```python
from build123d import *

# Parameters (mm, degrees)
SKETCH_1_W                         = 60
SKETCH_1_H                         = 20
SM_BASE_FLANGE_1_DEPTH             = 2
SM_EDGE_FLANGE_1_STRIP_W           = 13.4732
SM_EDGE_FLANGE_1_STRIP_H           = 2
SM_EDGE_FLANGE_1_STRIP_CUT_DEPTH   = 20
SM_EDGE_FLANGE_1_STRIP_2_W         = 13.4732
SM_EDGE_FLANGE_1_STRIP_2_H         = 2
SM_EDGE_FLANGE_1_STRIP_CUT_2_DEPTH = 20
SM_EDGE_FLANGE_1_DEPTH             = 20
SM_EDGE_FLANGE_1_BEND_DEPTH        = 20
SM_EDGE_FLANGE_1_PROFILE_W         = 45
SM_EDGE_FLANGE_1_PROFILE_H         = 17.2634
SM_EDGE_FLANGE_1_FLAT_DEPTH        = 2
RIB_2_REACH                        = 74.312
SKETCH_12_WALL_W                   = 160.765785142
SKETCH_12_WALL_H                   = 3
CUT_EXTRUDE_1_REACH                = 86.433
SKETCH_13_R                        = 2.75
CUT_EXTRUDE_1_DIRECTION_2_DEPTH    = 85.433405711
SKETCH_15_R                        = 2.75
CUT_EXTRUDE_2_DEPTH                = 10
SKETCH_16_R                        = 2.25
CUT_EXTRUDE_3_DEPTH                = 10


# Sheet-metal steps are written as plain solids
with BuildPart() as part:
    # Sketch 1 → 基体-法兰1 (new body)
    with BuildSketch(Plane(origin=(0, 0, 0), x_dir=(1, 0, 0), z_dir=(0, 1, 0))):
        Rectangle(SKETCH_1_W, SKETCH_1_H)
    extrude(amount=-SM_BASE_FLANGE_1_DEPTH)

    # 边线-法兰1 strip (across the edge) → 边线-法兰1 strip cut (cut)
    with BuildSketch(Plane(origin=(30, 0, 10), x_dir=(-1, 0, 0), z_dir=(0, 0, -1))):
        with Locations((-2, -1)):
            Rectangle(SM_EDGE_FLANGE_1_STRIP_W, SM_EDGE_FLANGE_1_STRIP_H)
    extrude(amount=SM_EDGE_FLANGE_1_STRIP_CUT_DEPTH, mode=Mode.SUBTRACT)

    # 边线-法兰1 strip 2 (across the edge) → 边线-法兰1 strip cut 2 (cut)
    with BuildSketch(Plane(origin=(-30, 0, -10), x_dir=(1, 0, 0), z_dir=(0, 0, 1))):
        with Locations((-2, -1)):
            Rectangle(SM_EDGE_FLANGE_1_STRIP_2_W, SM_EDGE_FLANGE_1_STRIP_2_H)
    extrude(amount=SM_EDGE_FLANGE_1_STRIP_CUT_2_DEPTH, mode=Mode.SUBTRACT)

    # 边线-法兰1 section (across the edge) → 边线-法兰1 (add)
    with BuildSketch(Plane(origin=(30, 0, 10), x_dir=(-1, 0, 0), z_dir=(0, 0, -1))):
        with BuildLine():
            Line((0, 2.7366), (0, 48))
            Line((0, 48), (2, 48))
            Line((2, 48), (2, 2.7366))
            ThreePointArc((2, 2.7366), (2.801531583, 0.801531583), (4.7366, 0))
            Line((4.7366, 0), (4.7366, -2))
            ThreePointArc((4.7366, -2), (1.38731802, -0.61268198), (0, 2.7366))
        make_face()
    extrude(amount=SM_EDGE_FLANGE_1_DEPTH)

    # 边线-法兰1 bend section (across the edge) → 边线-法兰1 bend (add)
    with BuildSketch(Plane(origin=(-30, 0, -10), x_dir=(1, 0, 0), z_dir=(0, 0, 1))):
        with BuildLine():
            Line((0, 2.7366), (2, 2.7366))
            ThreePointArc((2, 2.7366), (2.801531583, 0.801531583), (4.7366, 0))
            Line((4.7366, 0), (4.7366, -2))
            ThreePointArc((4.7366, -2), (1.38731802, -0.61268198), (0, 2.7366))
        make_face()
    extrude(amount=SM_EDGE_FLANGE_1_BEND_DEPTH)

    # 边线-法兰1 profile (on flange) → 边线-法兰1 flat (add)
    with BuildSketch(Plane(origin=(-30, 0, 0), x_dir=(0, 0, -1), z_dir=(1, 0, 0))):
        with Locations((-12.5, 11.3683)):
            Rectangle(SM_EDGE_FLANGE_1_PROFILE_W, SM_EDGE_FLANGE_1_PROFILE_H)
    extrude(amount=SM_EDGE_FLANGE_1_FLAT_DEPTH)

    # 草图12 wall → 筋2 (add, up to next)
    with BuildSketch(Plane(origin=(-23, 5, -10), x_dir=(0.707106781187, -0.707106781187, 0), z_dir=(-0.707106781187, -0.707106781187, 0)), mode=Mode.PRIVATE) as rib_2_sk1:
        with Locations((0, 1.5)):
            Rectangle(SKETCH_12_WALL_W, SKETCH_12_WALL_H)
    rib_2_tool1 = extrude(rib_2_sk1.sketch, amount=RIB_2_REACH, mode=Mode.PRIVATE) - part.part
    rib_2 = rib_2_tool1.solids().sort_by_distance((-23, 5, -10))[0]
    add(rib_2)

    # 镜向1: 筋2 across plane
    add(rib_2.mirror(Plane(origin=(0, 0, 0), x_dir=(0, 0, 1), z_dir=(1, 0, 0))))

    # 草图13 → 切除-拉伸1 (cut, up to next)
    with BuildSketch(Plane.ZY.offset(30), mode=Mode.PRIVATE) as cut_extrude_1_sk1:
        with Locations(Location((0, 13, 0), (0, 0, 90))):
            Circle(SKETCH_13_R)
    cut_extrude_1_tool1 = extrude(cut_extrude_1_sk1.sketch, amount=-CUT_EXTRUDE_1_REACH, mode=Mode.PRIVATE) & part.part
    # 草图13 → 切除-拉伸1 (cut, up to next)
    with BuildSketch(Plane.ZY.offset(30), mode=Mode.PRIVATE) as cut_extrude_1_sk2:
        with Locations(Location((19, 13, 0), (0, 0, 90))):
            Circle(SKETCH_13_R)
    cut_extrude_1_tool2 = extrude(cut_extrude_1_sk2.sketch, amount=-CUT_EXTRUDE_1_REACH, mode=Mode.PRIVATE) & part.part
    # 草图13 → 切除-拉伸1 (cut, up to next)
    with BuildSketch(Plane.ZY.offset(30), mode=Mode.PRIVATE) as cut_extrude_1_sk3:
        with Locations(Location((30, 13, 0), (0, 0, 90))):
            Circle(SKETCH_13_R)
    cut_extrude_1_tool3 = extrude(cut_extrude_1_sk3.sketch, amount=-CUT_EXTRUDE_1_REACH, mode=Mode.PRIVATE) & part.part
    add(cut_extrude_1_tool1.solids().sort_by_distance((-30, 13, 0))[0], mode=Mode.SUBTRACT)
    add(cut_extrude_1_tool2.solids().sort_by_distance((-30, 13, 19))[0], mode=Mode.SUBTRACT)
    add(cut_extrude_1_tool3.solids().sort_by_distance((-30, 13, 30))[0], mode=Mode.SUBTRACT)

    # 草图13 → 切除-拉伸1 direction 2 (cut)
    with BuildSketch(Plane.ZY.offset(30)):
        with Locations(Location((0, 13, 0), (0, 0, 90))):
            Circle(SKETCH_13_R)
        with Locations(Location((19, 13, 0), (0, 0, 90))):
            Circle(SKETCH_13_R)
        with Locations(Location((30, 13, 0), (0, 0, 90))):
            Circle(SKETCH_13_R)
    extrude(amount=CUT_EXTRUDE_1_DIRECTION_2_DEPTH, mode=Mode.SUBTRACT)

    # 草图15 → 切除-拉伸2 (cut)
    with BuildSketch(Plane.ZY.offset(-28)):
        with Locations(Location((-5.5, 21, 0), (0, 0, 270))):
            Circle(SKETCH_15_R)
        with Locations(Location((5.5, 21, 0), (0, 0, 270))):
            Circle(SKETCH_15_R)
        with Locations(Location((5.5, 41, 0), (0, 0, 270))):
            Circle(SKETCH_15_R)
        with Locations(Location((-5.5, 41, 0), (0, 0, 270))):
            Circle(SKETCH_15_R)
    extrude(amount=-CUT_EXTRUDE_2_DEPTH, mode=Mode.SUBTRACT)

    # 草图16 → 切除-拉伸3 (cut)
    with BuildSketch(Plane.XZ.offset(2)):
        with Locations(Location((9.593773501, 0, 0), (0, 0, 270))):
            Circle(SKETCH_16_R)
        with Locations(Location((-6.30510484, 0, 0), (0, 0, 270))):
            Circle(SKETCH_16_R)
    extrude(amount=-CUT_EXTRUDE_3_DEPTH, mode=Mode.SUBTRACT)


solid = part.part
```
Check sheet for the modelled part. Datum: model origin and axes. Units: mm. A direction names the side the tool comes from. Coordinates: 2 decimals unless noted, no trailing zeros. Order: outer loops, then holes, each group sorted by start corner. A loop starts at its lowest first (then second) coordinate and runs counter-clockwise, first axis right, second up. Notation, with made-up numbers: (-9, -16) -> (11, -16) arc R24 cw to (11, 12) -> close; hole circle Ø3 at (66.5, -13.75). An arc over 180 degrees is marked (long way). Write item = value, one per line. Start each with the question number.
1) Cross-section at A-A (y = 21). Enter the section's corners in (x, z), then the cut area to 3 significant figures.
2) Cross-section at C-C (z = 5.5). Enter the section's corners in (x, y), then the cut area to 3 significant figures.
3) Mould release check, pull along Z, two halves, no side actions. Record for faces 1 (the flat face through (-29, 20, 13)), 2 (the flat face through (1, -0.2, -10)), 3 (the cylindrical face through (28.986, 23.747, 5.621)), 4 (the cylindrical face through (28.986, 43.747, -5.379)): +Z half, -Z half, draft (parallel to the pull), parting line (faces both ways), or undercut.
4) Material ranges on L1, parallel to Z at x = -29.6, y = 13; L2, parallel to Z at x = 28.5, y = 41; L3, parallel to X at y = 16.5, z = -2, recorded low to high.
5) Cross-section at B-B (y = 13). Enter the section's corners in (x, z), then the cut area to 3 significant figures.
6) Cross-section at D-D (z = 19). Enter the section's corners in (x, y).
7) Access from +Z, -Z, +X, -X, +Y, -Y to the whole of each face (thin tool, end or side, straight path). Record for faces 5 (the cylindrical face through (28.986, 23.747, -5.379)), 6 (the flat face through (-28, 11, 13)), 7 (the flat face through (23, 5, -8)), 8 (the flat face through (-29, 2.737, 23)).
8) Go/stop test with flat-tipped pins: P1, Ø5, axis at x = 1, z = 6.5, coming from the +Y side; P2, Ø12, axis at x = 19, y = 9, coming from the +Z side; P3, Ø9, axis at y = 41, z = -5.5, coming from the -X side; P4, Ø7, axis at y = 21, z = 5.5, coming from the -X side. Record where each tip stops, or that it passes through.
Ans:
q1.outline = (28, -10) -> (30, -10) -> (30, -8.25) -> (28, -8.25) -> close; (28, -2.75) -> (30, -2.75) -> (30, 2.75) -> (28, 2.75) -> close; (28, 8.25) -> (30, 8.25) -> (30, 10) -> (28, 10) -> close
q1.area = 18.0 mm²
q2.outline = (-30, 2.74) arc R4.74 ccw to (-25.26, -2) -> (25.26, -2) arc R4.74 ccw to (30, 2.74) -> (30, 18.25) -> (28, 18.25) -> (28, 2.74) arc R2.74 cw to (25.26, 0) -> (-25.26, 0) arc R2.74 cw to (-28, 2.74) -> (-28, 20) -> (-30, 20) -> close; (28, 23.75) -> (30, 23.75) -> (30, 38.25) -> (28, 38.25) -> close; (28, 43.75) -> (30, 43.75) -> (30, 48) -> (28, 48) -> close
q2.area = 228 mm²
q3.face_1 = draft
q3.face_2 = -Z half
q3.face_3 = undercut
q3.face_4 = undercut
q4.L1 = -10 to -2.75, 2.75 to 16.25, 21.75 to 27.25, 32.75 to 35
q4.L2 = -10 to -8.25, -2.75 to 2.75, 8.25 to 10
q4.L3 = -30 to -28, 28 to 30
q5.outline = (-30, -10) -> (-28, -10) -> (-28, -2.75) -> (-30, -2.75) -> close; (-30, 2.75) -> (-28, 2.75) -> (-28, 16.25) -> (-30, 16.25) -> close; (-30, 21.75) -> (-28, 21.75) -> (-28, 27.25) -> (-30, 27.25) -> close; (-30, 32.75) -> (-28, 32.75) -> (-28, 35) -> (-30, 35) -> close; (28, -10) -> (30, -10) -> (30, 10) -> (28, 10) -> close
q5.area = 97.0 mm²
q6.outline = (-30, 2.74) -> (-28, 2.74) -> (-28, 10.25) -> (-30, 10.25) -> close; (-30, 15.75) -> (-28, 15.75) -> (-28, 20) -> (-30, 20) -> close
q7.face_5 = +X
q7.face_6 = +Z, +Y
q7.face_7 = +Z, -Z, +Y
q7.face_8 = +Z, +X, -X, -Y
q8.P1 = 0
q8.P2 = -7
q8.P3 = 28
q8.P4 = -30
